Input: part model. Units: mm. Frame: model coordinates. A direction names the side the tool comes from. Round coordinates to 2 decimals unless told otherwise and drop trailing zeros. Loops run counter-clockwise (first coordinate to the right, second up) from the corner with the lowest first, then second, coordinate; pieces in that order, holes last.
(1) Cut plane B-B, the plane y = 19.05. Output: boundary loops of the cut face in (x, z).
(2) First-contact query: pin 1 Ø8 at (x, y) = (31.75, 19.05) entering from -Z; pin 2 Ø6 at (y, z) = (-7.5, -30) entering from -X; pin 3 Ø5 at (y, z) = (-4.5, 14.5) entering from -X; pin 4 Ø8 at (x, z) = (3.5, -16) entering from +Y. Flat tips, straight axial feed; report the tip coordinate or a pass-through.
(3) Cut plane A-A, the plane x = 0. Output: boundary loops of the cut face in (y, z), and give its area (3 significant figures).
(4) Cut plane D-D, the plane x = -11.5. Output: boundary loops of the cut face in (y, z).
(5) Draft query along X for faces 1 (the face through (31.079, 24.162, 31.839)), 2 (the face through (-44.45, -6, 13)), 3 (the face through (-0.671, -6.439, -26.638)), 4 (the face through (50.8, 12, 32)). Return one class per face: released by +X, released by -X, zero draft, split by the parting line, or undercut.
(6) Access query for faces 5 (the face through (9, 0, -11)), 6 (the face through (44.45, -6, 13)), 7 (the face through (-1, 15, 38.1)). Directions: +Z, -Z, +X, -X, +Y, -Y. A direction counts if a zero-diameter tool reaches every point of the face in a straight line with its end or side. Return the directions, or none.
(7) Line query: line 1 (Z direction, x = 0, y = -4.25); line 2 (Y direction, x = 27, z = 16); line 3 (Z direction, x = 2.5, y = 27). Output: solid intervals per line, ascending.
(8) Cut plane C-C, the plane z = -31.75. Output: boundary loops of the cut face in (x, y).
from build123d import *

# Parameters (mm, degrees)
F1_DEPTH = 12.7
F2_W     = 101.6
F2_H     = 50.8
F3_DEPTH = 12.7
F4_R     = 12.68349
F5_DEPTH = 25.4
F6_R     = 5.1562
F7_DEPTH = 25.4
F8_R     = 5.1562
F9_DEPTH = 25.4
F10_R    = 3.81


with BuildPart() as f1:
    # F0 (on Front) → F1 (new body)
    with BuildSketch(Plane.XZ):
        with BuildLine():
            Line((-44.45, 25.4), (-44.45, 0))
            ThreePointArc((-44.45, 0), (0, -44.45), (44.45, 0))
            Line((44.45, 0), (44.45, 25.4))
            Line((44.45, 25.4), (-44.45, 25.4))
        make_face()
    extrude(amount=F1_DEPTH)

    # F2 (on face) → F3 (join)
    with BuildSketch(Plane.XY.offset(25.4)):
        with Locations((0, 12.7)):
            Rectangle(F2_W, F2_H)
    extrude(amount=F3_DEPTH)

    # F4 (on face) → F5 (cut)
    with BuildSketch(Plane.XZ.offset(12.7)):
        Circle(F4_R)
    extrude(amount=-F5_DEPTH, mode=Mode.SUBTRACT)

    # F6 (on face) → F7 (cut)
    with BuildSketch(Plane.XZ.offset(12.7)):
        with Locations((0, -31.75)):
            Circle(F6_R)
        with Locations((-31.75, 0)):
            Circle(F6_R)
        with Locations((31.75, 0)):
            Circle(F6_R)
    extrude(amount=-F7_DEPTH, mode=Mode.SUBTRACT)

    # F8 (on face) → F9 (cut)
    with BuildSketch(Plane.XY.offset(38.1)):
        with Locations((-31.75, 19.05)):
            Circle(F8_R)
        with Locations((31.75, 19.05)):
            Circle(F8_R)
    extrude(amount=-F9_DEPTH, mode=Mode.SUBTRACT)

    # F10
    f10_edges = [f1.edges().sort_by_distance(p)[0] for p in [
        (0, 0, 25.4),
        (0, -12.7, 38.1),
    ]]
    fillet(f10_edges, radius=F10_R)


solid = f1.part
Reported:
1. outline: (-50.8, 25.4) - (-36.91, 25.4) - (-36.91, 38.1) - (-50.8, 38.1) - close; (-26.59, 25.4) - (26.59, 25.4) - (26.59, 38.1) - (-26.59, 38.1) - close; (36.91, 25.4) - (50.8, 25.4) - (50.8, 38.1) - (36.91, 38.1) - close
2. pin 1: passes through
2. pin 2: stops at x = -35.31
2. pin 3: stops at x = -44.45
2. pin 4: stops at y = 0
3. outline: (-12.7, -44.45) - (0, -44.45) - (0, -36.91) - (-12.7, -36.91) - close; (-12.7, -26.59) - (0, -26.59) - (0, -12.68) - (-12.7, -12.68) - close; (-12.7, 12.68) - (0, 12.68) - (0, 21.59) arc R3.81 cw to (3.81, 25.4) - (38.1, 25.4) - (38.1, 38.1) - (-8.89, 38.1) arc R3.81 ccw to (-12.7, 34.29) - close
3. area: 1,080 mm2
4. outline: (-12.7, -42.94) - (0, -42.94) - (0, -5.35) - (-12.7, -5.35) - close; (-12.7, 5.35) - (0, 5.35) - (0, 21.59) arc R3.81 cw to (3.81, 25.4) - (38.1, 25.4) - (38.1, 38.1) - (-8.89, 38.1) arc R3.81 ccw to (-12.7, 34.29) - close
5. face 1: undercut
5. face 2: released by -X
5. face 3: undercut
5. face 4: released by +X
6. face 5: -Z, +X, -X, +Y
6. face 6: -Z, +X, +Y, -Y
6. face 7: +Z, +X, -X, +Y, -Y
7. line 1: z = -44.45 to -36.91, -26.59 to -12.68, 12.68 to 38.1
7. line 2: y = -12.7 to 0
7. line 3: z = 25.4 to 38.1
8. outline: (-31.11, -12.7) - (-5.16, -12.7) - (-5.16, 0) - (-31.11, 0) - close; (5.16, -12.7) - (31.11, -12.7) - (31.11, 0) - (5.16, 0) - close
